The model under review builds one solid part; all positions refer to its coordinate system, in mm. Face numbers are marked on the shaded views. A direction names the side the tool comes from. Coordinates: 2 decimals unless noted, no trailing zeros. Order: outer loops, then holes, each group sorted by start corner. A loop starts at its lowest first (then second) coordinate and runs counter-clockwise, first axis right, second up.
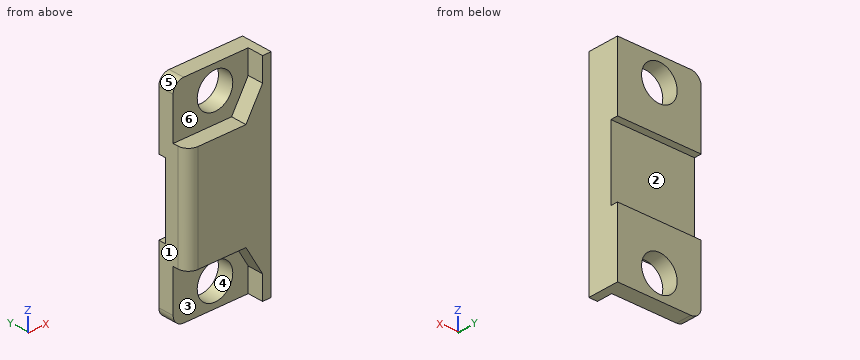
```python
from build123d import *

# Parameters (mm, degrees)
CROQUIS1_W              = 8
CROQUIS1_H              = 20
CROQUIS1_R              = 1.7
SALIENTE_EXTRUIR1_DEPTH = 3
CORTAR_EXTRUIR2_DEPTH   = 1.5
CORTAR_EXTRUIR3_REACH   = 25.601
CROQUIS3_W              = 7
CROQUIS3_H              = 1
REDONDEO1_R             = 1
CROQUIS4_W              = 8
CROQUIS4_H              = 7
SALIENTE_EXTRUIR2_DEPTH = 0.3


with BuildPart() as part:
    # Croquis1 → Saliente-Extruir1 (new body)
    with BuildSketch(Plane(origin=(0, 0, 0), x_dir=(1, 0, 0), z_dir=(0, 1, 0))):
        with Locations((165.962302832, -11.999998776)):
            Rectangle(CROQUIS1_W, CROQUIS1_H)
        with Locations(Location((165.962302832, -4.249998776, 0), (0, 0, 270))):
            Circle(CROQUIS1_R, mode=Mode.SUBTRACT)
        with Locations(Location((165.962302832, -19.75, 0), (0, 0, 270))):
            Circle(CROQUIS1_R, mode=Mode.SUBTRACT)
    extrude(amount=-SALIENTE_EXTRUIR1_DEPTH)

    # Croquis2 → Cortar-Extruir2 (cut)
    with BuildSketch(Plane.XZ.offset(3)):
        Polygon((164.374589592, 17), (167.550016072, 17), (169.137729313, 19.75), (169.137729313, 21.999998776), (161.962302832, 21.999998776), (161.962302832, 17), align=None)
        Polygon((161.962302832, 6.999997552), (164.374589592, 6.999997552), (167.550016072, 6.999997552), (169.137729313, 4.249997552), (169.137729313, 1.999998776), (161.962302832, 1.999998776), align=None)
    extrude(amount=-CORTAR_EXTRUIR2_DEPTH, mode=Mode.SUBTRACT)

    # Croquis3 → Cortar-Extruir3 (cut, up to next)
    with BuildSketch(Plane.ZY.offset(-161.962302832), mode=Mode.PRIVATE) as cortar_extruir3_sk1:
        with Locations((11.999998776, -0.5)):
            Rectangle(CROQUIS3_W, CROQUIS3_H)
    cortar_extruir3_tool1 = extrude(cortar_extruir3_sk1.sketch, amount=-CORTAR_EXTRUIR3_REACH, mode=Mode.PRIVATE) & part.part
    add(cortar_extruir3_tool1.solids().sort_by_distance((161.962303, -0.5, 11.999999))[0], mode=Mode.SUBTRACT)

    # Redondeo1
    redondeo1_edges = [part.edges().sort_by_distance(p)[0] for p in [
        (161.962302832, -0.75, 21.999998776),
        (161.962302832, -3, 11.999998776),
        (161.962302832, -0.75, 1.999998776),
    ]]
    fillet(redondeo1_edges, radius=REDONDEO1_R)

    # Croquis4 → Saliente-Extruir2 (add)
    with BuildSketch(Plane(origin=(0, -1, 0), x_dir=(1, 0, 0), z_dir=(0, 1, 0))):
        with Locations((165.962302832, -11.999998776)):
            Rectangle(CROQUIS4_W, CROQUIS4_H)
    extrude(amount=SALIENTE_EXTRUIR2_DEPTH)


solid = part.part
```
(1) Wall thickness on probe 1 along Z at (x, y) = (165.5, -0.3); probe 2 along Z at (x, y) = (165, -0.8); probe 3 along Z at (x, y) = (165.5, -0.9): over which ranges is each line inside the solid? List them lowest first.
A:
probe 1: z = 2 to 2.61, 5.89 to 8.5, 15.5 to 18.11, 21.39 to 22
probe 2: z = 2 to 2.85, 5.65 to 18.35, 21.15 to 22
probe 3: z = 2 to 2.61, 5.89 to 18.11, 21.39 to 22
(2) For pin 1 Ø1 at (x, z) = (166.5, 18.5) entering from -Y; pin 2 Ø1.6 at (x, y) = (164, -2.5) entering from -Z; pin 3 Ø0.8 at (y, z) = (-2, 3.5) entering from -X, all flat-tipped, find the tip position at first contact; note any pin that passes through.
A:
pin 1: stops at y = -1.5
pin 2: stops at z = 7
pin 3: stops at x = 169.14
(3) Machinability: for the marked faces 1, 2 and 3, which of the approach directions +Z, -Z, +X, -X, +Y, -Y give a long, thin tool a straight path to every point of the face, cutting with its end or side? Answer none if there is none.
A:
face 1: +Z, -Z, -X, +Y, -Y
face 2: +X, -X, +Y
face 3: -Z, -X, -Y
(4) We need section A-A, the plane x = 166.5. Write out the cut boundary in (y, z).
A:
outline: (-3, 7) - (-1.5, 7) - (-1.5, 5.86) - (0, 5.86) - (0, 8.5) - (-0.7, 8.5) - (-0.7, 15.5) - (0, 15.5) - (0, 18.14) - (-1.5, 18.14) - (-1.5, 17) - (-3, 17) - close; (-1.5, 2) - (0, 2) - (0, 2.64) - (-1.5, 2.64) - close; (-1.5, 21.36) - (0, 21.36) - (0, 22) - (-1.5, 22) - close
(5) Draft analysis for pull direction X (two halves, no side actions). For the marked faces 4, 5 and 6, state which applies: released by +X, released by -X, zero draft, split by the parting line, or undercut.
A:
face 4: undercut
face 5: released by -X
face 6: zero draft
(6) We need section B-B, the plane y = -1.1. Write out the cut boundary in (x, z), and give its area (3 significant figures).
A:
outline: (161.96, 3) arc R1 ccw to (162.96, 2) - (169.96, 2) - (169.96, 22) - (162.96, 22) arc R1 ccw to (161.96, 21) - close; hole circle Ø3.4 at (165.96, 4.25); hole circle Ø3.4 at (165.96, 19.75)
area: 141 mm2
(7) We need section D-D, the plane x = 162.75. Write out the cut boundary in (y, z), and give its area (3 significant figures).
A:
outline: (-2.98, 7) - (-1.5, 7) - (-1.5, 2.02) - (0, 2.02) - (0, 8.5) - (-0.7, 8.5) - (-0.7, 15.5) - (0, 15.5) - (0, 21.98) - (-1.5, 21.98) - (-1.5, 17) - (-2.98, 17) - close
area: 39.8 mm2
(8) We need section C-C, the plane z = 11.25. Write out the cut boundary in (x, y).
A:
outline: (161.96, -2) arc R1 ccw to (162.96, -3) - (169.96, -3) - (169.96, -0.7) - (161.96, -0.7) - close
